The drawing under review shows one solid part. Ordinate dimensions are in mm from its lowest x, y, z. A direction names the side the tool comes from. Give positions to 0.01 mm unless a question says otherwise; leave off trailing zeros. Write each loop counter-clockwise with the first axis right and the second up, starting at its lowest first coordinate (ties: lowest second). Pieces come first, ordered by that corner, then holes. Notation, with made-up numbers: M 74.25,20.25 L 133.25,20.25 A27 cw 133.25,52.25 Z; hole C 19,15.5 d1. An arc over 180 degrees is marked long. Use one line per item in the form item = value. Start each with the question number.
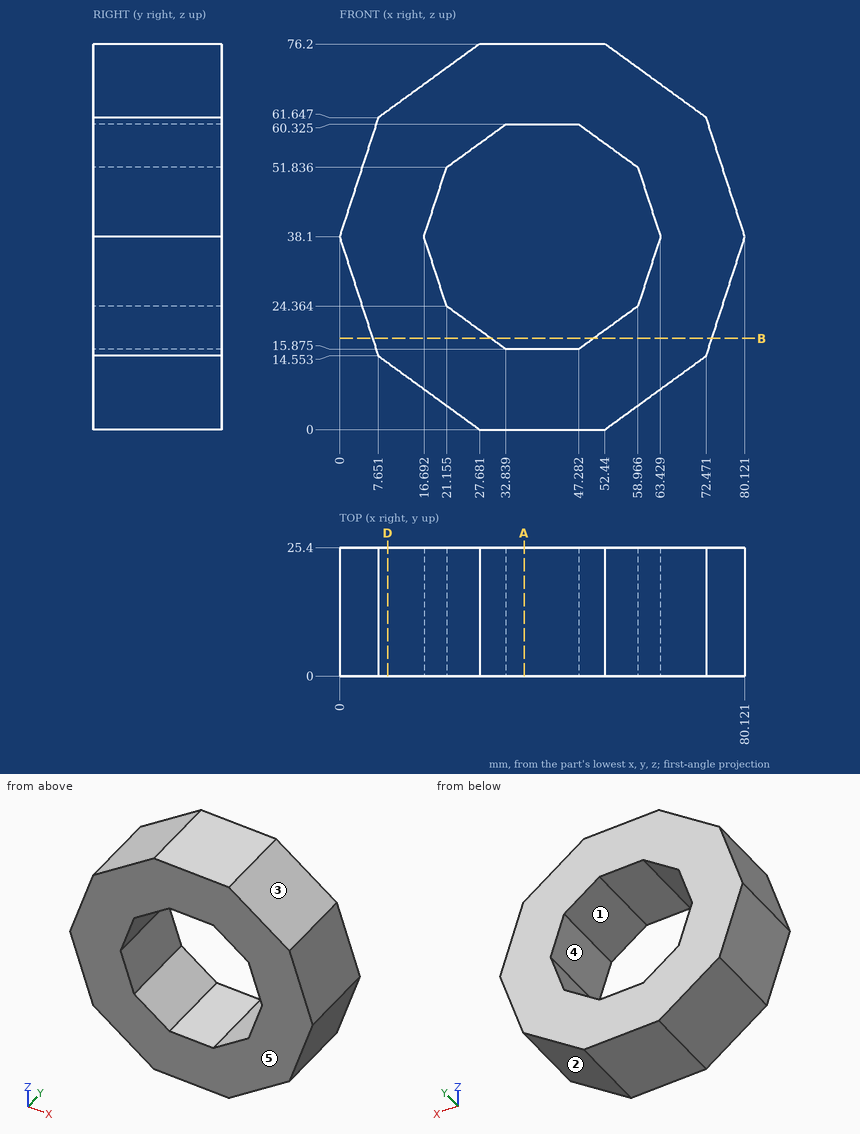
1. We need section A-A (x = 36.5). State the section outline as (y, z) points (1 decimal).
2. We need section B-B (z = 18). State the section outline as (x, y) points (1 decimal).
3. Clearance check with flat-ended pins moving along their axes: pin 1 Ø5 at (y, z) = (17.5, 14) entering from +X; pin 2 Ø12 at (y, z) = (9, 44) entering from +X; pin 3 Ø4 at (y, z) = (8.5, 54.5) entering from -X; pin 4 Ø5 at (y, z) = (20.5, 49.5) entering from +X. State where each tip first meets the part, or that it passes through.
4. Draft analysis for pull direction Z (two halves, no side actions). For the marked faces 3, 4 and 5, state which applies: pulls with the +Z half, pulls with the -Z half, needs draft (parallel to the pull), parting line crosses it, or undercut.
5. To check wall thickness, follow L1, parallel to Z at x = 42.5, y = 19.5 (1 decimal); L2, parallel to X at y = 14.75, z = 34 (1 decimal); L3, parallel to Z at x = 57.5, y = 17 (1 decimal). State the ranges of each line that lie inside material, in increasing order.
6. For the marked faces 1 and 2, list the 3-axis set-ups (+Z, -Z, +X, -X, +Y, -Y) from which the entire face can be reached by the end or side of a thin tool; tool diameter is ignored.
7. We need section D-D (x = 9.5). State the section outline as (y, z) points, and give its area (3 significant figures).
Answer block:
q1.outline = M 0,0 L 25.4,0 L 25.4,15.9 L 0,15.9 Z; M 0,60.3 L 25.4,60.3 L 25.4,76.2 L 0,76.2 Z
q2.outline = M 6.5,0 L 29.9,0 L 29.9,25.4 L 6.5,25.4 Z; M 50.2,0 L 73.6,0 L 73.6,25.4 L 50.2,25.4 Z
q3.pin_1 = 73.1
q3.pin_2 = 80.12
q3.pin_3 = 4.68
q3.pin_4 = 77.23
q4.face_3 = pulls with the +Z half
q4.face_4 = undercut
q4.face_5 = needs draft
q5.L1 = 0 to 15.9, 60.3 to 76.2
q5.L2 = 1.3 to 18, 62.1 to 78.8
q5.L3 = 3.7 to 23.3, 52.9 to 72.5
q6.face_1 = +Y, -Y
q6.face_2 = -Z, +X, +Y, -Y
q7.outline = M 0,13.21 L 25.4,13.21 L 25.4,62.99 L 0,62.99 Z
q7.area = 1,260 mm^2
